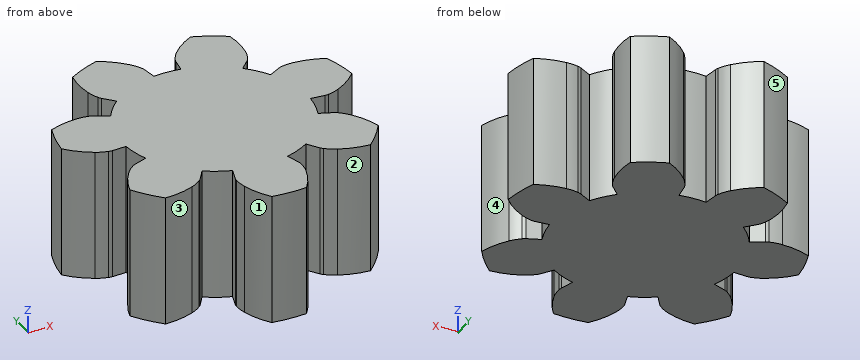
Autodesk Inventor part; units mm, degrees
ref_plane "YZ Plane" through (0, 0, 0) normal (1, 0, 0) x (0, 1, 0)
ref_plane "XZ Plane" through (0, 0, 0) normal (0, 1, 0) x (-1, 0, 0)
ref_plane "XY Plane" through (0, 0, 0) normal (0, 0, 1) x (1, 0, 0)
sketch "Sketch1" plane through (0, 0, 0) normal (0, 0, 1) x (1, 0, 0)
  arc A0 (0.5156, 3.3554) -> (0.4821, 3.2534) centre (0.9432, 3.1583) ccw
  arc A1 (0.7215, 3.6793) -> (0.5156, 3.3554) centre (1.7274, 2.8124) ccw
  arc A2 (1.4571, 4.2576) -> (0.7215, 3.6793) centre (2.5636, 2.0932) ccw
  arc A3 (-2.3019, 2.4952) -> (-2.2431, 2.4054) centre (-1.8812, 2.7066) ccw
  arc A4 (-2.4267, 2.8581) -> (-2.3019, 2.4952) centre (-1.1218, 3.104) ccw
  arc A5 (-2.4202, 3.7937) -> (-2.4267, 2.8581) centre (-0.0382, 3.3094) ccw
  arc A6 (-3.386, -0.244) -> (-3.2791, -0.254) centre (-3.289, 0.2168) ccw
  arc A7 (-3.7476, -0.1153) -> (-3.386, -0.244) centre (-3.1262, 1.0583) ccw
  arc A8 (-4.4751, 0.4731) -> (-3.7476, -0.1153) centre (-2.6112, 2.0335) ccw
  arc A9 (-1.9204, -2.7994) -> (-1.8459, -2.7221) centre (-2.2201, -2.4363) ccw
  arc A10 (-2.2464, -3.0019) -> (-1.9204, -2.7994) centre (-2.7766, -1.7844) ccw
  arc A11 (-3.1601, -3.2037) -> (-2.2464, -3.0019) centre (-3.2179, -0.7736) ccw
  arc A12 (0.9913, -3.2468) -> (0.9773, -3.1404) centre (0.5205, -3.2548) ccw
  arc A13 (0.9463, -3.628) -> (0.9913, -3.2468) centre (-0.3361, -3.2833) ccw
  arc A14 (0.5345, -4.4681) -> (0.9463, -3.628) centre (-1.4015, -2.9982) ccw
  arc A15 (3.1566, -1.2493) -> (3.0646, -1.1939) centre (2.8692, -1.6223) ccw
  arc A16 (3.4265, -1.5221) -> (3.1566, -1.2493) centre (2.3575, -2.3099) ccw
  arc A17 (3.8266, -2.3679) -> (3.4265, -1.5221) centre (1.4703, -2.9651) ccw
  arc A18 (2.9448, 1.689) -> (2.8442, 1.6516) centre (3.0573, 1.2317) ccw
  arc A19 (3.3264, 1.7299) -> (2.9448, 1.689) centre (3.2758, 0.4029) ccw
  arc A20 (4.2372, 1.5154) -> (3.3264, 1.7299) centre (3.2349, -0.6992) ccw
  arc A21 (-0.4821, 3.2534) -> (-0.5156, 3.3554) centre (-0.9432, 3.1583) ccw
  arc A22 (-0.5156, 3.3554) -> (-0.7215, 3.6793) centre (-1.7274, 2.8124) ccw
  arc A23 (-0.7215, 3.6793) -> (-1.4571, 4.2576) centre (-2.5636, 2.0932) ccw
  arc A24 (-2.8442, 1.6516) -> (-2.9448, 1.689) centre (-3.0573, 1.2317) ccw
  arc A25 (-2.9448, 1.689) -> (-3.3264, 1.7299) centre (-3.2758, 0.4029) ccw
  arc A26 (-3.3264, 1.7299) -> (-4.2372, 1.5154) centre (-3.2349, -0.6992) ccw
  arc A27 (-3.0646, -1.1939) -> (-3.1566, -1.2493) centre (-2.8692, -1.6223) ccw
  arc A28 (-3.1566, -1.2493) -> (-3.4265, -1.5221) centre (-2.3575, -2.3099) ccw
  arc A29 (-3.4265, -1.5221) -> (-3.8266, -2.3679) centre (-1.4703, -2.9651) ccw
  arc A30 (-0.9773, -3.1404) -> (-0.9913, -3.2468) centre (-0.5205, -3.2548) ccw
  arc A31 (-0.9913, -3.2468) -> (-0.9463, -3.628) centre (0.3361, -3.2833) ccw
  arc A32 (-0.9463, -3.628) -> (-0.5345, -4.4681) centre (1.4015, -2.9982) ccw
  arc A33 (1.8459, -2.7221) -> (1.9204, -2.7994) centre (2.2201, -2.4363) ccw
  arc A34 (1.9204, -2.7994) -> (2.2464, -3.0019) centre (2.7766, -1.7844) ccw
  arc A35 (2.2464, -3.0019) -> (3.1601, -3.2037) centre (3.2179, -0.7736) ccw
  arc A36 (3.2791, -0.254) -> (3.386, -0.244) centre (3.289, 0.2168) ccw
  arc A37 (3.386, -0.244) -> (3.7476, -0.1153) centre (3.1262, 1.0583) ccw
  arc A38 (3.7476, -0.1153) -> (4.4751, 0.4731) centre (2.6112, 2.0335) ccw
  arc A39 (2.2431, 2.4054) -> (2.3019, 2.4952) centre (1.8812, 2.7066) ccw
  arc A40 (2.3019, 2.4952) -> (2.4267, 2.8581) centre (1.1218, 3.104) ccw
  arc A41 (2.4267, 2.8581) -> (2.4202, 3.7937) centre (0.0382, 3.3094) ccw
  arc A42 (0.4177, 2.8192) -> (-0.4177, 2.8192) centre (0, 0) ccw
  arc A43 (-1.9437, 2.0843) -> (-2.4646, 1.4312) centre (0, 0) ccw
  arc A44 (-2.8415, -0.2201) -> (-2.6556, -1.0346) centre (0, 0) ccw
  arc A45 (-1.5996, -2.3588) -> (-0.8469, -2.7213) centre (0, 0) ccw
  arc A46 (0.8469, -2.7213) -> (1.5996, -2.3588) centre (0, 0) ccw
  arc A47 (2.6556, -1.0346) -> (2.8415, -0.2201) centre (0, 0) ccw
  arc A48 (2.4646, 1.4312) -> (1.9437, 2.0843) centre (0, 0) ccw
  arc A49 (-1.4571, 4.2576) -> (-2.4202, 3.7937) centre (0, 0) ccw
  arc A50 (-4.2372, 1.5154) -> (-4.4751, 0.4731) centre (0, 0) ccw
  arc A51 (-3.8266, -2.3679) -> (-3.1601, -3.2037) centre (0, 0) ccw
  arc A52 (-0.5345, -4.4681) -> (0.5345, -4.4681) centre (0, 0) ccw
  arc A53 (3.1601, -3.2037) -> (3.8266, -2.3679) centre (0, 0) ccw
  arc A54 (4.4751, 0.4731) -> (4.2372, 1.5154) centre (0, 0) ccw
  arc A55 (2.4202, 3.7937) -> (1.4571, 4.2576) centre (0, 0) ccw
  line L0 (0.4177, 2.8192) -> (0.4821, 3.2534)
  line L1 (-1.9437, 2.0843) -> (-2.2431, 2.4054)
  line L2 (-2.8415, -0.2201) -> (-3.2791, -0.254)
  line L3 (-1.5996, -2.3588) -> (-1.8459, -2.7221)
  line L4 (0.8469, -2.7213) -> (0.9773, -3.1404)
  line L5 (2.6556, -1.0346) -> (3.0646, -1.1939)
  line L6 (2.4646, 1.4312) -> (2.8442, 1.6516)
  line L7 (-0.4177, 2.8192) -> (-0.4821, 3.2534)
  line L8 (-2.4646, 1.4312) -> (-2.8442, 1.6516)
  line L9 (-2.6556, -1.0346) -> (-3.0646, -1.1939)
  line L10 (-0.8469, -2.7213) -> (-0.9773, -3.1404)
  line L11 (1.5996, -2.3588) -> (1.8459, -2.7221)
  line L12 (2.8415, -0.2201) -> (3.2791, -0.254)
  line L13 (1.9437, 2.0843) -> (2.2431, 2.4054)
extrude "Extrusion1" add sketch "Sketch1" against normal blind 4
properties part number "初段多段部分歯数7"
Here's how the part is built. I have some questions about the finished solid (model axes, mm). Face numbers are marked on the shaded views. A direction names the side the tool comes from. Round coordinates to 2 decimals unless told otherwise and drop trailing zeros. Write each loop counter-clockwise with the first axis right and the second up, starting at its lowest first coordinate (ties: lowest second). Pieces come first, ordered by that corner, then holes.
Q1. Please list where these lines run through material, in increasing order: probe 1 along X at (y, z) = (-3, -3); probe 2 along X at (y, z) = (-3.5, -2.7); probe 3 along Y at (x, z) = (0, -0.55).
Q2. If we section it at A-A on y = -2: Write out the boundary of the cut face in (x, z).
Q3. If we section it at B-B on x = -0.25: Write out the boundary of the cut face in (y, z), plus the area to 3 significant figures.
Q4. If we mould it in two halves opening along X, with no side actions, what happens to the marked faces 3, 4 and 5? For each: +X half, -X half, draft (parallel to the pull), parting line (faces both ways), or undercut.
Q5. Which directions (+Z, -Z, +X, -X, +Y, -Y) give clear straight access to the entire face, cutting with the end or side of a thin tool? Please do the marked faces 1 and 2.
Answer below:
1. probe 1: x = -3.35 to -2.24, -0.93 to 0.93, 2.24 to 3.35
1. probe 2: x = -0.97 to 0.97
1. probe 3: y = -4.5 to 2.85
2. outline: (-3.7, -4) - (3.7, -4) - (3.7, 0) - (-3.7, 0) - close
3. outline: (-4.49, -4) - (2.84, -4) - (2.84, 0) - (-4.49, 0) - close
3. area: 29.3 mm2
4. face 3: undercut
4. face 4: +X half
4. face 5: -X half
5. face 1: +Z, -Z, -X, -Y
5. face 2: +Z, -Z, -Y
